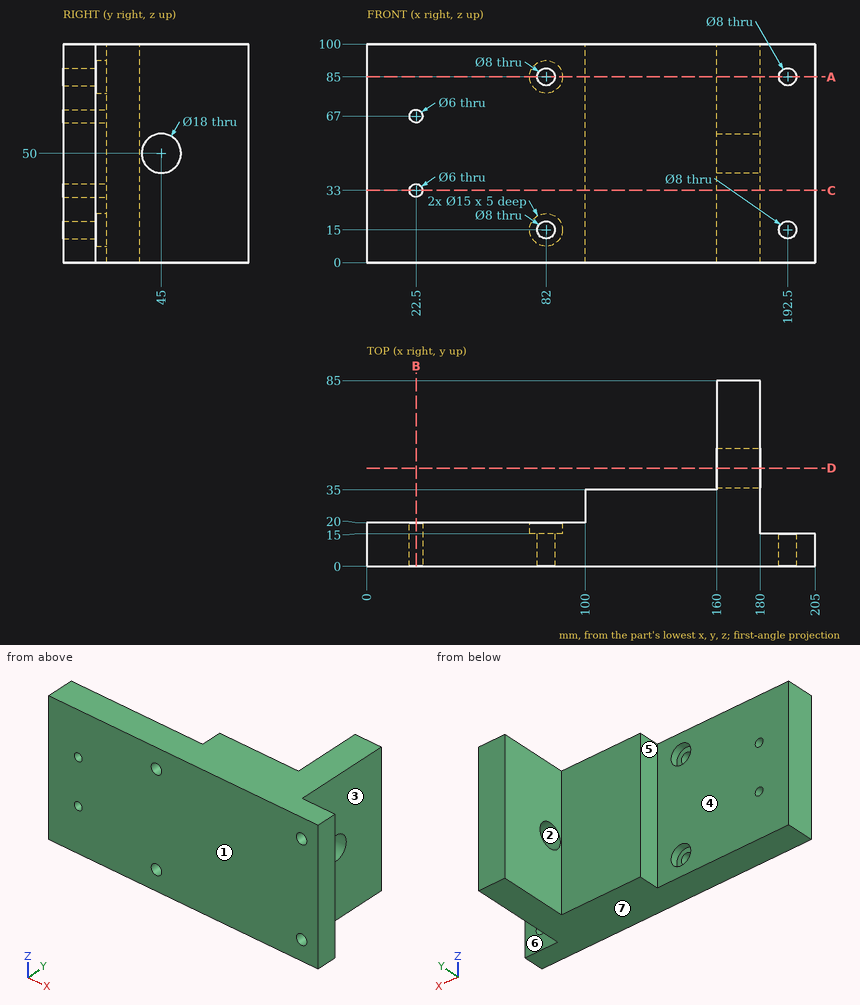
Here's the drawing with two shaded views (mm, measured from the low corner). I have some questions. A direction names the side the tool comes from. Round coordinates to 2 decimals unless told otherwise and drop trailing zeros. Loops run counter-clockwise (first coordinate to the right, second up) from the corner with the lowest first, then second, coordinate; pieces in that order, holes last. Notation, with made-up numbers: M 33,38 L 72,38 A26 cw 72,63 Z; hole C 81.25,81 d6. An arc over 180 degrees is marked long. Put each result on its own line as item: value.
Q1. For pin 1 (7.5 mm diameter, centred on x = 84.5, z = 85, fed in from +Y); pin 2 (4.5 mm diameter, centred on y = 26, z = 54, fed in from -X); pin 3 (1 mm diameter, centred on x = 122.5, z = 70, fed in from +Y), each with a flat end and sliding along its axis, tell me the tip position at first contact or that it passes through.
Check result:
pin 1: y = 15
pin 2: x = 100
pin 3: y = 35
Q2. On a 3-axis mill with a long thin cutter (end or side, diameter ignored), from which of +Z, -Z, +X, -X, +Y, -Y can I reach the whole of each face in a straight line? I mean the marked faces 5, 6 and 7. Say none if no direction works.
Check result:
face 5: +Z, -Z, -X, +Y
face 6: +Z, -Z, +X, +Y
face 7: -Z, +X, -X, +Y, -Y
Q3. I need wall thicknesses on probe 1 along Z at (x, y) = (82, 18.05); probe 2 along Y at (x, z) = (174, 50); probe 3 along X at (y, z) = (15.5, 67). Which ranges of each line are inside material? Lowest first, please.
Check result:
probe 1: 0 to 7.5, 22.5 to 77.5, 92.5 to 100
probe 2: 0 to 36, 54 to 85
probe 3: 0 to 19.5, 25.5 to 180
Q4. Imagine slicing it at C-C (z = 33). Write out the boundary of the cut face in (x, y), then the cut area to 4 significant figures.
Check result:
outline: M 0,0 L 19.5,0 L 19.5,20 L 0,20 Z; M 25.5,0 L 205,0 L 205,15 L 180,15 L 180,85 L 160,85 L 160,35 L 100,35 L 100,20 L 25.5,20 Z
area: 6,055 mm2
Q5. Imagine slicing it at B-B (x = 22.5). Write out the boundary of the cut face in (y, z), then the cut area to 3 significant figures.
Check result:
outline: M 0,0 L 20,0 L 20,30 L 0,30 Z; M 0,36 L 20,36 L 20,64 L 0,64 Z; M 0,70 L 20,70 L 20,100 L 0,100 Z
area: 1,760 mm2
Q6. Thinking about a two-plate mould opening in Y: for the marked faces 1, 2, 3 and 4, which applies, released by +Y, released by -Y, zero draft, split by the parting line, or undercut?
Check result:
face 1: released by -Y
face 2: undercut
face 3: zero draft
face 4: released by +Y
Q7. Imagine slicing it at A-A (z = 85). Write out the boundary of the cut face in (x, y), then the cut area to 3 significant figures.
Check result:
outline: M 0,0 L 78,0 L 78,15 L 74.5,15 L 74.5,20 L 0,20 Z; M 86,0 L 188.5,0 L 188.5,15 L 180,15 L 180,85 L 160,85 L 160,35 L 100,35 L 100,20 L 89.5,20 L 89.5,15 L 86,15 Z; M 196.5,0 L 205,0 L 205,15 L 196.5,15 Z
area: 5,860 mm2
Q8. Imagine slicing it at D-D (y = 45). Write out the boundary of the cut face in (x, z), then the cut area to 3 significant figures.
Check result:
outline: M 160,0 L 180,0 L 180,41 L 160,41 Z; M 160,59 L 180,59 L 180,100 L 160,100 Z
area: 1,640 mm2
